Design review of the part built by this model. Coordinates are the model's own, in mm. Face numbers are marked on the shaded views. A direction names the side the tool comes from. Round coordinates to 2 decimals unless told otherwise and drop trailing zeros. Write each loop counter-clockwise with the first axis right and the second up, starting at its lowest first coordinate (ties: lowest second). Pieces come first, ordered by that corner, then holes. Notation, with made-up numbers: (18.5, 4) -> (69.5, 4) arc R13 ccw to (69.5, 26) -> close; hole circle Ø3 at (17, -12). An arc over 180 degrees is marked (long way). Write item = value, one per line. Start each with the question number.
Item 1: Add section A-A, the plane z = 0. State the section outline as (x, y) points, then the cut area to 3 significant figures.
Item 2: To check wall thickness, follow L1, parallel to X at y = 14.75, z = 0; L2, parallel to X at y = 55, z = -4; L3, parallel to X at y = 31, z = -21.5. State the ranges of each line that lie inside material, in increasing order.
Item 3: Add section C-C, the plane x = 41.5. State the section outline as (y, z) points.
Item 4: Add section B-B, the plane y = 40.5. State the section outline as (x, z) points, then the cut area to 3 significant figures.
Item 5: For pin 1 Ø2 at (x, y) = (-2, 16.5) entering from +Z; pin 2 Ø2 at (x, z) = (93.5, -14) entering from +Y; pin 3 Ø8 at (x, z) = (61.5, 23.5) entering from +Y; pin 4 Ø20 at (x, z) = (114, 0) entering from +Y, all flat-tipped, find the tip position at first contact; note any pin that passes through.
Item 6: Mouldability with a two-part tool opening along X and no side actions: class the marked faces 4, 5, 6 and 7 as released by +X, released by -X, zero draft, split by the parting line, or undercut.
Item 7: Machinability: for the marked faces 1, 2 and 3, which of the approach directions +Z, -Z, +X, -X, +Y, -Y give a long, thin tool a straight path to every point of the face, cutting with its end or side? Answer none if there is none.
Item 8: Add section D-D, the plane z = -24.5. State the section outline as (x, y) points, then the cut area to 3 significant figures.
from build123d import *

# Parameters (mm, degrees)
SKETCH1_R           = 11
BOSS_EXTRUDE1_DEPTH = 19
SKETCH2_W           = 64
SKETCH2_H           = 64
BOSS_EXTRUDE2_DEPTH = 45
CUT_EXTRUDE2_START  = -13
CUT_EXTRUDE2_DEPTH  = 45


with BuildPart() as part:
    # Sketch1 → Boss-Extrude1 (new body)
    with BuildSketch(Plane(origin=(0, 0, 0), x_dir=(1, 0, 0), z_dir=(0, 1, 0))):
        with BuildLine():
            Line((0, 32), (114, 32))
            ThreePointArc((114, 32), (146, 0), (114, -32))
            Line((114, -32), (0, -32))
            ThreePointArc((0, -32), (-32, 0), (0, 32))
        make_face()
        with Locations(Location((0, 0, 0), (0, 0, 270))):
            Circle(SKETCH1_R, mode=Mode.SUBTRACT)
        with Locations(Location((114, 0, 0), (0, 0, 270))):
            Circle(SKETCH1_R, mode=Mode.SUBTRACT)
    extrude(amount=BOSS_EXTRUDE1_DEPTH)

    # Sketch2 → Boss-Extrude2 (add)
    with BuildSketch(Plane(origin=(0, 19, 0), x_dir=(1, 0, 0), z_dir=(0, 1, 0))):
        with Locations((57, 0)):
            Rectangle(SKETCH2_W, SKETCH2_H)
    extrude(amount=BOSS_EXTRUDE2_DEPTH)

    # Sketch3 → Cut-Extrude2 (cut)
    with BuildSketch(Plane.ZY.offset(-25).offset(CUT_EXTRUDE2_START)):
        Polygon((32, 64), (-19, 64), (32, 13), align=None)
    extrude(amount=-CUT_EXTRUDE2_DEPTH, mode=Mode.SUBTRACT)


solid = part.part
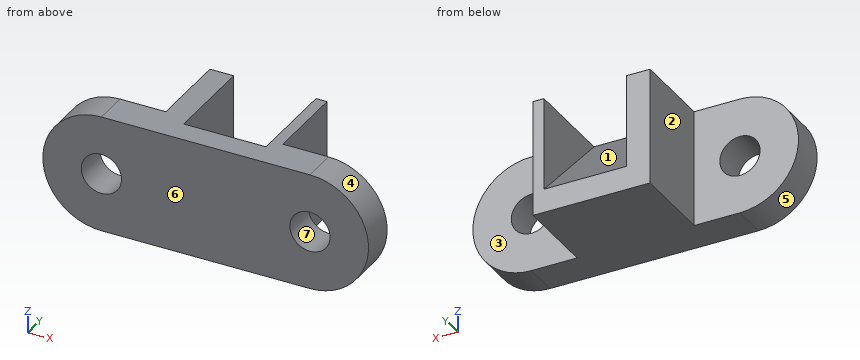
Result set:
q1.outline = (-32, 0) -> (-11, 0) -> (-11, 19) -> (-32, 19) -> close; (11, 0) -> (103, 0) -> (103, 19) -> (89, 19) -> (89, 64) -> (83, 64) -> (83, 45) -> (38, 45) -> (38, 64) -> (25, 64) -> (25, 19) -> (11, 19) -> close; (125, 0) -> (146, 0) -> (146, 19) -> (125, 19) -> close
q1.area = 4,570 mm²
q2.L1 = -32 to -11, 11 to 103, 125 to 146
q2.L2 = 25 to 38, 83 to 89
q2.L3 = 25 to 89
q3.outline = (0, -32) -> (64, -32) -> (64, -19) -> (13, 32) -> (0, 32) -> close
q4.outline = (25, -32) -> (89, -32) -> (89, 32) -> (83, 32) -> (83, 4.5) -> (38, 4.5) -> (38, 32) -> (25, 32) -> close
q4.area = 2,860 mm²
q5.pin_1 = 31.98
q5.pin_2 = 19
q5.pin_3 = 25.5
q5.pin_4 = through
q6.face_4 = released by +X
q6.face_5 = released by -X
q6.face_6 = zero draft
q6.face_7 = undercut
q7.face_1 = +Z, +Y
q7.face_2 = +Z, -Z, -X, +Y
q7.face_3 = +Z, -Z, +X, +Y
q8.outline = (-20.59, 0) -> (134.59, 0) -> (134.59, 19) -> (89, 19) -> (89, 64) -> (25, 64) -> (25, 19) -> (-20.59, 19) -> close
q8.area = 5,830 mm²
